For this review, take the finished solid that the model builds, in its own axes (mm). Round coordinates to 2 decimals unless told otherwise and drop trailing zeros. Order: outer loops, then holes, each group sorted by start corner. A loop starts at its lowest first (then second) coordinate and runs counter-clockwise, first axis right, second up. Notation, with made-up numbers: (-30.5, 8) -> (-17.5, 8) arc R14 ccw to (-17.5, 35) -> close; hole circle Ø3 at (-16, 56.25). An arc over 180 degrees is marked (long way). Answer in a Markdown table with one row per item.
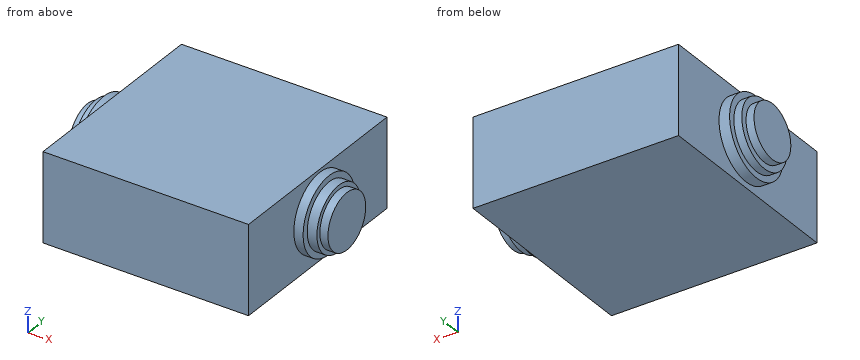
```python
from build123d import *

# Parameters (mm, degrees)
F0_W      = 154.612802
F0_H      = 154.072925
F1_DEPTH  = 66.8
F2_R      = 28.811278
F3_DEPTH  = 7
F4_R      = 24.288847
F5_DEPTH  = 7.3
F6_R      = 21.010708
F7_DEPTH  = 6.1
F8_R      = 29.852046
F9_DEPTH  = 8
F10_R     = 25.172837
F11_DEPTH = 6
F12_R     = 20.49857
F13_DEPTH = 6


with BuildPart() as f1:
    # F0 (on Top) → F1 (new body)
    with BuildSketch(Plane.XY):
        with Locations((2.452422, -2.169334)):
            Rectangle(F0_W, F0_H)
    extrude(amount=F1_DEPTH)

    # F2 (on face) → F3 (join)
    with BuildSketch(Plane.YZ.offset(79.758823)):
        with Locations((0, 35.756472)):
            Circle(F2_R)
    extrude(amount=F3_DEPTH)

    # F4 (on face) → F5 (join)
    with BuildSketch(Plane.YZ.offset(86.758823)):
        with Locations((0, 35.756472)):
            Circle(F4_R)
    extrude(amount=F5_DEPTH)

    # F6 (on face) → F7 (join)
    with BuildSketch(Plane.YZ.offset(94.058823)):
        with Locations((0, 35.756472)):
            Circle(F6_R)
    extrude(amount=F7_DEPTH)

    # F8 (on face) → F9 (join)
    with BuildSketch(Plane(origin=(-74.853979, 0, 0), x_dir=(0, -1, 0), z_dir=(-1, 0, 0))):
        with Locations((0, 34.220316)):
            Circle(F8_R)
    extrude(amount=F9_DEPTH)

    # F10 (on face) → F11 (join)
    with BuildSketch(Plane(origin=(-82.853979, 0, 0), x_dir=(0, -1, 0), z_dir=(-1, 0, 0))):
        with Locations((0, 34.220316)):
            Circle(F10_R)
    extrude(amount=F11_DEPTH)

    # F12 (on face) → F13 (join)
    with BuildSketch(Plane(origin=(-88.853979, 0, 0), x_dir=(0, -1, 0), z_dir=(-1, 0, 0))):
        with Locations((0, 34.220316)):
            Circle(F12_R)
    extrude(amount=F13_DEPTH)


solid = f1.part
```
Q1. Clearance check with flat-ended pins moving along their axes: pin 1 Ø10 at (y, z) = (-45.5, 43.5) entering from +X; pin 2 Ø12 at (y, z) = (-61.5, 32.5) entering from -X. State where each tip first meets the part, or that it passes through.
Answer key:
| item | result |
|---|---|
| pin 1 | stops at x = 79.76 |
| pin 2 | stops at x = -74.85 |
Q2. Take a section at A-A, the plane y = 0. Write out the cut boundary in (x, z), then the cut area to 3 significant figures.
Answer key:
| item | result |
|---|---|
| outline | (-94.85, 13.72) -> (-88.85, 13.72) -> (-88.85, 9.05) -> (-82.85, 9.05) -> (-82.85, 4.37) -> (-74.85, 4.37) -> (-74.85, 0) -> (79.76, 0) -> (79.76, 6.95) -> (86.76, 6.95) -> (86.76, 11.47) -> (94.06, 11.47) -> (94.06, 14.75) -> (100.16, 14.75) -> (100.16, 56.77) -> (94.06, 56.77) -> (94.06, 60.05) -> (86.76, 60.05) -> (86.76, 64.57) -> (79.76, 64.57) -> (79.76, 66.8) -> (-74.85, 66.8) -> (-74.85, 64.07) -> (-82.85, 64.07) -> (-82.85, 59.39) -> (-88.85, 59.39) -> (-88.85, 54.72) -> (-94.85, 54.72) -> close |
| area | 12,400 mm^2 |
Q3. Take a section at C-C, the plane y = -60. Write out the cut boundary in (x, z), then the cut area to 3 significant figures.
Answer key:
| item | result |
|---|---|
| outline | (-74.85, 0) -> (79.76, 0) -> (79.76, 66.8) -> (-74.85, 66.8) -> close |
| area | 10,300 mm^2 |
Q4. Take a section at B-B, the plane y = -17. Write out the cut boundary in (x, z), then the cut area to 3 significant figures.
Answer key:
| item | result |
|---|---|
| outline | (-94.85, 22.77) -> (-88.85, 22.77) -> (-88.85, 15.65) -> (-82.85, 15.65) -> (-82.85, 9.68) -> (-74.85, 9.68) -> (-74.85, 0) -> (79.76, 0) -> (79.76, 12.5) -> (86.76, 12.5) -> (86.76, 18.41) -> (94.06, 18.41) -> (94.06, 23.41) -> (100.16, 23.41) -> (100.16, 48.1) -> (94.06, 48.1) -> (94.06, 53.1) -> (86.76, 53.1) -> (86.76, 59.02) -> (79.76, 59.02) -> (79.76, 66.8) -> (-74.85, 66.8) -> (-74.85, 58.76) -> (-82.85, 58.76) -> (-82.85, 52.79) -> (-88.85, 52.79) -> (-88.85, 45.67) -> (-94.85, 45.67) -> close |
| area | 11,800 mm^2 |
Q5. To check wall thickness, follow probe 1 along X at (y, z) = (-40, 33); probe 2 along X at (y, z) = (-23, 19); probe 3 along Y at (x, z) = (87, 16). State the ranges of each line that lie inside material, in increasing order.
Answer key:
| item | result |
|---|---|
| probe 1 | x = -74.85 to 79.76 |
| probe 2 | x = -82.85 to 86.76 |
| probe 3 | y = -14.13 to 14.13 |
